```python
from build123d import *

# Parameters (mm, degrees)
BASE_EXTR_DEPTH                                 = 5
MOTOR_1_EXTR_DEPTH                              = 41
SHAFT_MOTOR_SUPPORT_EXTR_DEPTH                  = 25
TAP_DRILL_FOR_M3X0_5_TAP1_D                     = 2.5
TAP_DRILL_FOR_M3X0_5_TAP1_DEPTH                 = 41
TAP_DRILL_FOR_M3X0_5_TAP1_TIP                   = 0.751075774
BOSS_EXTRUDE10_DEPTH                            = 20
CSK_FOR_M3_OVAL_HEAD_MACHINE_SCREW1_D           = 3.6
CSK_FOR_M3_OVAL_HEAD_MACHINE_SCREW1_DEPTH       = 14
CSK_FOR_M3_OVAL_HEAD_MACHINE_SCREW1_CSINK_D     = 6.3
CSK_FOR_M3_OVAL_HEAD_MACHINE_SCREW1_CSINK_ANGLE = 90
CSK_FOR_M3_OVAL_HEAD_MACHINE_SCREW1_TIP         = 1.081549114
CSK_FOR_M3_OVAL_HEAD_MACHINE_SCREW2_D           = 3.6
CSK_FOR_M3_OVAL_HEAD_MACHINE_SCREW2_DEPTH       = 14
CSK_FOR_M3_OVAL_HEAD_MACHINE_SCREW2_CSINK_D     = 6.3
CSK_FOR_M3_OVAL_HEAD_MACHINE_SCREW2_CSINK_ANGLE = 90
CSK_FOR_M3_OVAL_HEAD_MACHINE_SCREW2_TIP         = 1.081549114
TAP_DRILL_FOR_M3X0_5_TAP2_D                     = 2.5
TAP_DRILL_FOR_M3X0_5_TAP2_DEPTH                 = 14
TAP_DRILL_FOR_M3X0_5_TAP2_TIP                   = 0.751075774
TAP_DRILL_FOR_M3X0_5_TAP3_D                     = 2.5
TAP_DRILL_FOR_M3X0_5_TAP3_DEPTH                 = 14
TAP_DRILL_FOR_M3X0_5_TAP3_TIP                   = 0.751075774


with BuildPart() as part:
    # Base_sch → base_extr (new body)
    with BuildSketch(Plane(origin=(0, 0, 0), x_dir=(1, 0, 0), z_dir=(0, 1, 0))):
        Polygon((25, 10.5), (25, 25), (-25, 25), (-25, -25), (25, -25), (25, -10.5), (175, -10.5), (175, -25), (225.013827764, -25), (225.013827764, 25), (175, 25), (175, 10.5), align=None)
    extrude(amount=BASE_EXTR_DEPTH)

    # motor_support_sch → Motor_1_extr (add)
    with BuildSketch(Plane(origin=(0, 5, 0), x_dir=(1, 0, 0), z_dir=(0, 1, 0))):
        Polygon((-25, 16.439389634), (-25, 25), (-16.439389634, 25), (-16.439389634, 21), (-18.719694817, 18.719694817), (-21, 16.439389634), align=None)
        Polygon((16.439389634, 25), (25, 25), (25, 16.439389634), (21, 16.439389634), (18.719694817, 18.719694817), (16.439389634, 21), align=None)
        Polygon((25, -16.439389634), (25, -25), (16.439389634, -25), (16.439389634, -21), (18.719694817, -18.719694817), (21, -16.439389634), align=None)
        Polygon((-18.719694817, -18.719694817), (-21, -16.439389634), (-25, -16.439389634), (-25, -25), (-16.439389634, -25), (-16.439389634, -21), align=None)
    extrude(amount=MOTOR_1_EXTR_DEPTH)

    # shaft_motor_support_sch → shaft_motor_support_extr (add)
    with BuildSketch(Plane(origin=(0, 5, 0), x_dir=(1, 0, 0), z_dir=(0, 1, 0))):
        Polygon((181.280305183, -18.719694817), (179, -16.439389634), (175, -16.439389634), (175, -25), (183.560610366, -25), (183.560610366, -21), align=None)
        Polygon((175, 25), (175, 16.402508948), (179, 16.402508948), (183.560610366, 21.024047525), (183.560610366, 25), align=None)
        Polygon((225.013827764, -25), (225.013827764, -16.439389634), (221.056642929, -16.439389634), (216.38573482, -21), (216.38573482, -25), align=None)
        Polygon((225.013827764, 25), (216.38573482, 25), (216.38573482, 21.024047525), (221.056642929, 16.402508948), (225.013827764, 16.402508948), align=None)
    extrude(amount=SHAFT_MOTOR_SUPPORT_EXTR_DEPTH)

    # Tap Drill for M3x0.5 Tap1
    with Locations(Plane(origin=(0, 46, 0), x_dir=(1, 0, 0), z_dir=(0, 1, 0))):
        with Locations((-21, -21), (21, -21), (21, 21), (-21, 21), (179.013827764, 21), (221.013827764, 21), (221.013827764, -21), (179.013827764, -21)):
            Hole(TAP_DRILL_FOR_M3X0_5_TAP1_D / 2, depth=TAP_DRILL_FOR_M3X0_5_TAP1_DEPTH)
            with Locations((0, 0, -(TAP_DRILL_FOR_M3X0_5_TAP1_DEPTH + TAP_DRILL_FOR_M3X0_5_TAP1_TIP / 2))):  # 118° drill point
                Cone(0, TAP_DRILL_FOR_M3X0_5_TAP1_D / 2, TAP_DRILL_FOR_M3X0_5_TAP1_TIP, mode=Mode.SUBTRACT)

    # Sketch12 → Boss-Extrude10 (add)
    with BuildSketch(Plane.XZ):
        with BuildLine():
            Line((175, 25), (175, 55))
            Line((175, 55), (225.013827764, 55))
            Line((225.013827764, 55), (225.013827764, 41))
            Line((225.013827764, 41), (203.983092952, 41))
            ThreePointArc((203.983092952, 41), (195.906913882, 40), (203.983092952, 39))
            Line((203.983092952, 39), (225.013827764, 39))
            Line((225.013827764, 39), (225.013827764, 25))
            Line((225.013827764, 25), (175, 25))
        make_face()
        with BuildLine():
            Line((175, -25), (175, -55))
            Line((175, -55), (225.013827764, -55))
            Line((225.013827764, -55), (225.013827764, -41))
            Line((225.013827764, -41), (203.983092952, -41))
            ThreePointArc((203.983092952, -41), (195.906913882, -40), (203.983092952, -39))
            Line((203.983092952, -39), (225.013827764, -39))
            Line((225.013827764, -39), (225.013827764, -25))
            Line((225.013827764, -25), (175, -25))
        make_face()
    extrude(amount=-BOSS_EXTRUDE10_DEPTH)

    # CSK for M3 Oval Head Machine Screw1
    with Locations(Plane(origin=(220.013827764, 10, 55), x_dir=(1, 0, 0), z_dir=(0, 0, 1))):
        with Locations((0, 0)):
            CounterSinkHole(CSK_FOR_M3_OVAL_HEAD_MACHINE_SCREW1_D / 2, CSK_FOR_M3_OVAL_HEAD_MACHINE_SCREW1_CSINK_D / 2, depth=CSK_FOR_M3_OVAL_HEAD_MACHINE_SCREW1_DEPTH, counter_sink_angle=CSK_FOR_M3_OVAL_HEAD_MACHINE_SCREW1_CSINK_ANGLE)
            with Locations((0, 0, -(CSK_FOR_M3_OVAL_HEAD_MACHINE_SCREW1_DEPTH + CSK_FOR_M3_OVAL_HEAD_MACHINE_SCREW1_TIP / 2))):  # 118° drill point
                Cone(0, CSK_FOR_M3_OVAL_HEAD_MACHINE_SCREW1_D / 2, CSK_FOR_M3_OVAL_HEAD_MACHINE_SCREW1_TIP, mode=Mode.SUBTRACT)

    # CSK for M3 Oval Head Machine Screw2
    with Locations(Plane(origin=(220.013827764, 10, -55), x_dir=(-1, 0, 0), z_dir=(0, 0, -1))):
        with Locations((0, 0)):
            CounterSinkHole(CSK_FOR_M3_OVAL_HEAD_MACHINE_SCREW2_D / 2, CSK_FOR_M3_OVAL_HEAD_MACHINE_SCREW2_CSINK_D / 2, depth=CSK_FOR_M3_OVAL_HEAD_MACHINE_SCREW2_DEPTH, counter_sink_angle=CSK_FOR_M3_OVAL_HEAD_MACHINE_SCREW2_CSINK_ANGLE)
            with Locations((0, 0, -(CSK_FOR_M3_OVAL_HEAD_MACHINE_SCREW2_DEPTH + CSK_FOR_M3_OVAL_HEAD_MACHINE_SCREW2_TIP / 2))):  # 118° drill point
                Cone(0, CSK_FOR_M3_OVAL_HEAD_MACHINE_SCREW2_D / 2, CSK_FOR_M3_OVAL_HEAD_MACHINE_SCREW2_TIP, mode=Mode.SUBTRACT)

    # Tap Drill for M3x0.5 Tap2
    with Locations(Plane(origin=(0, 0, -39), x_dir=(-1, 0, 0), z_dir=(0, 0, -1))):
        with Locations((-220.013827764, 10)):
            Hole(TAP_DRILL_FOR_M3X0_5_TAP2_D / 2, depth=TAP_DRILL_FOR_M3X0_5_TAP2_DEPTH)
            with Locations((0, 0, -(TAP_DRILL_FOR_M3X0_5_TAP2_DEPTH + TAP_DRILL_FOR_M3X0_5_TAP2_TIP / 2))):  # 118° drill point
                Cone(0, TAP_DRILL_FOR_M3X0_5_TAP2_D / 2, TAP_DRILL_FOR_M3X0_5_TAP2_TIP, mode=Mode.SUBTRACT)

    # Tap Drill for M3x0.5 Tap3
    with Locations(Plane.XY.offset(39)):
        with Locations((220.013827764, 10)):
            Hole(TAP_DRILL_FOR_M3X0_5_TAP3_D / 2, depth=TAP_DRILL_FOR_M3X0_5_TAP3_DEPTH)
            with Locations((0, 0, -(TAP_DRILL_FOR_M3X0_5_TAP3_DEPTH + TAP_DRILL_FOR_M3X0_5_TAP3_TIP / 2))):  # 118° drill point
                Cone(0, TAP_DRILL_FOR_M3X0_5_TAP3_D / 2, TAP_DRILL_FOR_M3X0_5_TAP3_TIP, mode=Mode.SUBTRACT)


solid = part.part
```
Can you work these out from the model? Positions are in its coordinate system, mm. A direction names the side the tool comes from. Coordinates: 2 decimals unless noted, no trailing zeros. Loops run counter-clockwise (first coordinate to the right, second up) from the corner with the lowest first, then second, coordinate; pieces in that order, holes last.
Item 1: Which directions (+Z, -Z, +X, -X, +Y, -Y) give clear straight access to the entire face, cutting with the end or side of a thin tool? Please do faces 1 (the face through (25, 23, -21)), 2 (the face through (194, 20, -40)), 3 (the face through (218.75, 17.32, 18.69)), 4 (the face through (215, 10, -41)), 5 (the face through (178, 30, 20)).
Answers below:
face 1: -Z, +Y, -Y
face 2: -Z, +X, -X, +Y
face 3: +Y
face 4: +X, +Y, -Y
face 5: +Z, -Z, +X, +Y
Item 2: I'm going to push flat-ended pins straight in: pin 1 (2 mm diameter, centred on x = 221.01, z = -21, fed in from +Y); pin 2 (1.2 mm diameter, centred on y = 35.5, z = 22.5, fed in from +X); pin 3 (8 mm diameter, centred on x = 22.5, y = 20.5, fed in from +Z). Where does each tip first touch, or does it pass through?
Answers below:
pin 1: stops at y = 4.85
pin 2: stops at x = 25
pin 3: stops at z = 25
Item 3: Suppose I cut it at A-A (y = 35). Please give me the cut outline in (x, z), then the cut area to 3 significant figures.
Answers below:
outline: (-25, -25) - (-16.44, -25) - (-16.44, -21) - (-21, -16.44) - (-25, -16.44) - close; (-25, 16.44) - (-21, 16.44) - (-16.44, 21) - (-16.44, 25) - (-25, 25) - close; (16.44, -25) - (25, -25) - (25, -16.44) - (21, -16.44) - (16.44, -21) - close; (16.44, 21) - (21, 16.44) - (25, 16.44) - (25, 25) - (16.44, 25) - close; hole circle Ø2.5 at (-21, -21); hole circle Ø2.5 at (-21, 21); hole circle Ø2.5 at (21, -21); hole circle Ø2.5 at (21, 21)
area: 232 mm2
Item 4: Suppose I cut it at C-C (x = 192.5). Please give me the cut outline in (y, z).
Answers below:
outline: (0, -55) - (20, -55) - (20, -25) - (5, -25) - (5, 25) - (20, 25) - (20, 55) - (0, 55) - close
Item 5: Suppose I cut it at B-B (z = -14). Please give me the cut outline in (x, y).
Answers below:
outline: (-25, 0) - (25, 0) - (25, 5) - (-25, 5) - close; (175, 0) - (225.01, 0) - (225.01, 5) - (175, 5) - close
Item 6: If we mould it in two halves opening along Z, with no side actions, what happens to faces 6 (the face through (98, 5, 0)), 7 (the face through (180, 30, -22)), 8 (the face through (200, 10, -55))? For each: released by +Z, released by -Z, zero draft, split by the parting line, or undercut.
Answers below:
face 6: undercut
face 7: zero draft
face 8: released by -Z
Item 7: Please list where these lines run through material, in increasing order: L1, parallel to Z at x = 213.5, y = 13.5; L2, parallel to Z at x = 190, y = 18.5; L3, parallel to X at y = 30.5, z = -21.5.
Answers below:
L1: z = -55 to -41, -39 to -25, 25 to 39, 41 to 55
L2: z = -55 to -25, 25 to 55
L3: x = -25 to -22.15, -19.85 to -16.44, 16.44 to 19.85, 22.15 to 25
Item 8: Suppose I cut it at D-D (z = 27.5). Please give me the cut outline in (x, y), then the cut area to 3 significant figures.
Answers below:
outline: (175, 0) - (225.01, 0) - (225.01, 20) - (175, 20) - close; hole circle Ø2.5 at (220.01, 10)
area: 995 mm2
